```python
from build123d import *

# Parameters (mm, degrees)
F1_DEPTH = 76.2
F2_R     = 25.4
F3_DEPTH = 25.4


with BuildPart() as f1:
    # F0 (on Front) → F1 (new body)
    with BuildSketch(Plane.XZ):
        Polygon((-40.079643, -11.612137), (-40.079643, -37.012137), (36.120357, -37.012137), (36.120357, -11.612137), (10.720357, -11.612137), (10.720357, 51.887863), (36.120357, 51.887863), (36.120357, 77.287863), (-40.079643, 77.287863), (-40.079643, 51.887863), (-14.679643, 51.887863), (-14.679643, -11.612137), align=None)
    extrude(amount=F1_DEPTH)

    # F2 (on face) → F3 (cut)
    with BuildSketch(Plane.YZ.offset(10.720357)):
        with Locations((-38.1, 20.137863)):
            Circle(F2_R)
    extrude(amount=-F3_DEPTH, mode=Mode.SUBTRACT)


solid = f1.part
```
Can you work these out from the model? Positions are in its coordinate system, mm. A direction names the side the tool comes from. Coordinates: 2 decimals unless noted, no trailing zeros. Loops run counter-clockwise (first coordinate to the right, second up) from the corner with the lowest first, then second, coordinate; pieces in that order, holes last. Notation, with made-up numbers: (-38, -34.75) -> (-28, -34.75) arc R11 ccw to (-28, -19.75) -> close; hole circle Ø4 at (51, 25.25). An arc over 180 degrees is marked (long way). Put each result on its own line as item: value. Start each with the question number.
Q1. I want a section at A-A (x = -24). Write out the boundary of the cut face in (y, z), plus the area to 3 significant figures.
Q2. For faces 4 (the face through (10.72, -12, 20)), 5 (the face through (36.12, -38, -24)), 6 (the face through (-27, -38, -11.612)), which set-ups out of +Z, -Z, +X, -X, +Y, -Y let a thin tool reach every point of the face, with its end or its side?
Q3. I want a section at D-D (y = -72). Write out the boundary of the cut face in (x, z).
Q4. I want a section at B-B (y = -38.1). Write out the boundary of the cut face in (x, z).
Q5. I want a section at C-C (z = 42). Write out the boundary of the cut face in (x, y).
Q6. Thinking about a two-plate mould opening in Z: for faces 1 (the face through (-1, -38, 77.288)), 2 (the face through (-40.08, -38, -24)), 3 (the face through (24, -38, -11.612)), which applies, pulls with the +Z half, pulls with the -Z half, needs draft (parallel to the pull), parting line crosses it, or undercut?
Q7. If I drill on line 1 (Z direction, x = -6.5, y = -38.1); line 2 (Z direction, x = -17.5, y = -33); line 3 (X direction, y = -71, z = -9.5), over which ranges is the centre line in solid material (lowest first)? Write a range as [from, to].
Q8. I'm going to push a flat-ended pin straight in: P1, Ø1, axis at y = -22, z = 46, coming from the -X side. Where does the tip first touch, or does it pass through?
Taken from the geometry:
1. outline: (-76.2, -37.01) -> (0, -37.01) -> (0, -11.61) -> (-76.2, -11.61) -> close; (-76.2, 51.89) -> (0, 51.89) -> (0, 77.29) -> (-76.2, 77.29) -> close
1. area: 3,870 mm2
2. face 4: +X, +Y, -Y
2. face 5: +Z, -Z, +X, +Y, -Y
2. face 6: -X, +Y, -Y
3. outline: (-40.08, -37.01) -> (36.12, -37.01) -> (36.12, -11.61) -> (10.72, -11.61) -> (10.72, 51.89) -> (36.12, 51.89) -> (36.12, 77.29) -> (-40.08, 77.29) -> (-40.08, 51.89) -> (-14.68, 51.89) -> (-14.68, -11.61) -> (-40.08, -11.61) -> close
4. outline: (-40.08, -37.01) -> (36.12, -37.01) -> (36.12, -11.61) -> (10.72, -11.61) -> (10.72, -5.26) -> (-14.68, -5.26) -> (-14.68, -11.61) -> (-40.08, -11.61) -> close; (-40.08, 51.89) -> (-14.68, 51.89) -> (-14.68, 45.54) -> (10.72, 45.54) -> (10.72, 51.89) -> (36.12, 51.89) -> (36.12, 77.29) -> (-40.08, 77.29) -> close
5. outline: (-14.68, -76.2) -> (10.72, -76.2) -> (10.72, -51.03) -> (-14.68, -51.03) -> close; (-14.68, -25.17) -> (10.72, -25.17) -> (10.72, 0) -> (-14.68, 0) -> close
6. face 1: pulls with the +Z half
6. face 2: needs draft
6. face 3: undercut
7. line 1: z = [-37.01, -5.26], [45.54, 77.29]
7. line 2: z = [-37.01, -11.61], [51.89, 77.29]
7. line 3: x = [-14.68, 10.72]
8. P1: stops at x = -14.68
